Build history of the part. All positions in model axes, mm. A direction names the side the tool comes from. Give positions to 0.01 mm unless a question says otherwise; leave off trailing zeros. Order: outer loops, then holes, each group sorted by start corner. A loop starts at its lowest first (then second) coordinate and runs counter-clockwise, first axis right, second up. Notation, with made-up numbers: (79.5, -23) - (96.5, -23) arc R10 cw to (96.5, -9) - close; hole circle Ø7 at (62.25, 40). An arc over 180 degrees is marked (long way). Use a Markdown table: item, result. Add a question column.
(1) Flat gauge pins, fed straight in: pin 1 (4 mm diameter, centred on x = -3.5, z = -1.5, fed in from +Y); pin 2 (15 mm diameter, centred on x = 0, y = 96.25, fed in from -Z); pin 3 (0.8 mm diameter, centred on x = 5.5, y = -54.5, fed in from -Z). Where does each tip first touch, or does it go through?
(2) Wall check: line 1 (Y direction, x = 5, z = 3.5); line 2 (Y direction, x = 0, z = -0.55); line 3 (X direction, y = -102.25, z = 5). Give the ranges that are in metal, low to high.
(3) Slice it at A-A (y = -31.5). Write the cut outline in (x, z).
(4) Slice it at B-B (y = 93). Write the cut outline in (x, z).
(5) Mould opens along X. For faces 5 (the face through (18, -12, 17)), 6 (the face through (-6.5, 91, 6)), 7 (the face through (0, 113, 0)), 8 (the face through (0, 7, 19)) say: +X half, -X half, draft (parallel to the pull), parting line (faces both ways), or undercut.
(6) Which spindle directions (+Z, -Z, +X, -X, +Y, -Y) get a long thin tool onto all of the face, cutting with end or side? Do faces 1 (the face through (-13.594, -49.031, 15.056)), 2 (the face through (6.5, 91, 6)), 3 (the face through (0, -77, -2)), 4 (the face through (0.266, 70.219, 14.564)). Say none if no direction does.
from build123d import *

# Parameters (mm, degrees)
SKETCH1_W               = 38
SKETCH1_H               = 227.5
SKETCH1_W_2             = 21
SKETCH1_H_2             = 41
BOSS_EXTRUDE1_DEPTH     = 11
SKETCH3_R               = 1.3
CUT_EXTRUDE1_DEPTH      = 8
FILLET3_R               = 19
BOSS_EXTRUDE2_DEPTH     = 8
CUT_EXTRUDE2_DEPTH      = 117.880547997
CUT_EXTRUDE2_DEPTH_BACK = 117.880547997
SKETCH7_W               = 32
SKETCH7_H               = 157.5
BOSS_EXTRUDE4_DEPTH     = 8
SKETCH8_W               = 38
SKETCH8_H               = 157.5
BOSS_EXTRUDE5_DEPTH     = 8
BOSS_EXTRUDE10_START    = 2
SKETCH27_R              = 9
BOSS_EXTRUDE10_DEPTH    = 2
SKETCH28_W              = 38
SKETCH28_H              = 27
BOSS_EXTRUDE11_DEPTH    = 20
FILLET4_R               = 19
CUT_EXTRUDE14_DEPTH     = 8
SKETCH30_W              = 13
SKETCH30_H              = 24
CUT_EXTRUDE15_DEPTH     = 11
CUT_EXTRUDE16_REACH     = 138.422
SKETCH31_R              = 6.5
CUT_EXTRUDE17_START     = 65.75
CUT_EXTRUDE17_OUTLINE_W = 38
CUT_EXTRUDE17_OUTLINE_H = 6
CUT_EXTRUDE17_DEPTH     = 68
FILLET5_R               = 12
CUT_EXTRUDE18_DEPTH     = 141.335535414
FILLET7_R               = 5
SKETCH34_R              = 1.5
CUT_EXTRUDE19_DEPTH     = 8
SKETCH35_R              = 1.1
CUT_EXTRUDE20_DEPTH     = 8
FILLET8_R               = 8
SKETCH36_W              = 21
SKETCH36_H              = 40
CUT_EXTRUDE21_DEPTH     = 2


# Read off the part's stored shape, not the designer's step: Cut-Extrude17
# Some blends are built 0.0001 mm under size
with BuildPart() as part:
    # Sketch1 → Boss-Extrude1 (new body)
    with BuildSketch(Plane.XY):
        Rectangle(SKETCH1_W, SKETCH1_H)
        with Locations((0, -78.25)):
            Rectangle(SKETCH1_W_2, SKETCH1_H_2, mode=Mode.SUBTRACT)
    extrude(amount=BOSS_EXTRUDE1_DEPTH)

    # Sketch3 → Cut-Extrude1 (cut)
    with BuildSketch(Plane.XY.offset(10)):
        with Locations((-5, -54.25)):
            Circle(SKETCH3_R)
        with Locations((5, -54.25)):
            Circle(SKETCH3_R)
        with Locations((5, -102.25)):
            Circle(SKETCH3_R)
        with Locations((-5, -102.25)):
            Circle(SKETCH3_R)
    extrude(amount=-CUT_EXTRUDE1_DEPTH, mode=Mode.SUBTRACT)

    # Fillet3
    fillet3_edges = [part.edges().sort_by_distance(p)[0] for p in [
        (19, -113.75, 5.5),
        (-19, -113.75, 5.5),
    ]]
    fillet(fillet3_edges, radius=FILLET3_R - 0.0001)  # a hair under: the kernel refuses the full size

    # Sketch4 → Boss-Extrude2 (add)
    with BuildSketch(Plane.XY.offset(11)):
        with BuildLine():
            Line((19, -94.75), (19, 113.75))
            Line((19, 113.75), (-19, 113.75))
            Line((-19, 113.75), (-19, -94.75))
            ThreePointArc((-19, -94.75), (-13.435028843, -108.185028843), (0, -113.75))
            ThreePointArc((0, -113.75), (13.435028843, -108.185028843), (19, -94.75))
        make_face()
        with BuildLine():
            Line((16, -94.75), (16, 110.75))
            Line((16, 110.75), (-16, 110.75))
            Line((-16, 110.75), (-16, -94.75))
            ThreePointArc((-16, -94.75), (-11.313708499, -106.063708499), (0, -110.75))
            ThreePointArc((0, -110.75), (11.313708499, -106.063708499), (16, -94.75))
        make_face(mode=Mode.SUBTRACT)
    extrude(amount=BOSS_EXTRUDE2_DEPTH)

    # Sketch6 → Cut-Extrude2 (cut, two sides: drawn at the far end of the back side and taken through both)
    with BuildSketch(Plane(origin=(0, 0, 0), x_dir=(0, 0, -1), z_dir=(1, 0, 0)).offset(-CUT_EXTRUDE2_DEPTH_BACK)):
        Polygon((-13, -113.75), (-16, -88.75), (-19, -73.75), (-19, -113.75), align=None)
    extrude(amount=CUT_EXTRUDE2_DEPTH + CUT_EXTRUDE2_DEPTH_BACK, mode=Mode.SUBTRACT)

    # Sketch7 → Boss-Extrude4 (add)
    with BuildSketch(Plane.XY.offset(11)):
        with Locations((0, 32)):
            Rectangle(SKETCH7_W, SKETCH7_H)
    extrude(amount=BOSS_EXTRUDE4_DEPTH)

    # Sketch8 → Boss-Extrude5 (add)
    with BuildSketch(Plane(origin=(0, 0, 0), x_dir=(-1, 0, 0), z_dir=(0, 0, -1))):
        with Locations((0, 35)):
            Rectangle(SKETCH8_W, SKETCH8_H)
    extrude(amount=BOSS_EXTRUDE5_DEPTH)

    # Sketch27 → Boss-Extrude10 (add)
    with BuildSketch(Plane(origin=(0, 0, 0), x_dir=(-1, 0, 0), z_dir=(0, 0, -1)).offset(BOSS_EXTRUDE10_START)):
        with BuildLine():
            Line((19, -94.75), (19, -43.75))
            Line((19, -43.75), (-19, -43.75))
            Line((-19, -43.75), (-19, -94.75))
            ThreePointArc((-19, -94.75), (-13.435028843, -108.185028843), (0, -113.75))
            ThreePointArc((0, -113.75), (13.435028843, -108.185028843), (19, -94.75))
        make_face()
        with Locations((0, -88.5)):
            Circle(SKETCH27_R, mode=Mode.SUBTRACT)
    extrude(amount=-BOSS_EXTRUDE10_DEPTH)

    # Sketch28 → Boss-Extrude11 (add)
    with BuildSketch(Plane(origin=(0, 113.75, 0), x_dir=(1, 0, 0), z_dir=(0, 1, 0))):
        with Locations((0, -5.5)):
            Rectangle(SKETCH28_W, SKETCH28_H)
    extrude(amount=BOSS_EXTRUDE11_DEPTH)

    # Fillet4
    fillet4_edges = [part.edges().sort_by_distance(p)[0] for p in [
        (-19, 133.75, 5.5),
        (19, 133.75, 5.5),
    ]]
    fillet(fillet4_edges, radius=FILLET4_R - 0.0001)  # a hair under: the kernel refuses the full size

    # Sketch29 → Cut-Extrude14 (cut)
    with BuildSketch(Plane(origin=(0, 0, -8), x_dir=(-1, 0, 0), z_dir=(0, 0, -1))):
        with BuildLine():
            Line((16, 66.75), (16, 114.75))
            ThreePointArc((16, 114.75), (11.313708499, 126.063708499), (0, 130.75))
            ThreePointArc((0, 130.75), (-11.313708499, 126.063708499), (-16, 114.75))
            Line((-16, 114.75), (-16, 66.75))
            Line((-16, 66.75), (16, 66.75))
        make_face()
    extrude(amount=-CUT_EXTRUDE14_DEPTH, mode=Mode.SUBTRACT)

    # Sketch30 → Cut-Extrude15 (cut)
    with BuildSketch(Plane(origin=(0, 0, 0), x_dir=(-1, 0, 0), z_dir=(0, 0, -1))):
        with Locations((0, 90.75)):
            Rectangle(SKETCH30_W, SKETCH30_H)
    extrude(amount=-CUT_EXTRUDE15_DEPTH, mode=Mode.SUBTRACT)

    # Sketch31 → Cut-Extrude16 (cut, up to next)
    with BuildSketch(Plane(origin=(0, 0, 11), x_dir=(-1, 0, 0), z_dir=(0, 0, -1)), mode=Mode.PRIVATE) as cut_extrude16_sk1:
        with Locations(Location((0, 96.25, 0), (0, 0, 180))):
            Circle(SKETCH31_R)
    cut_extrude16_tool1 = extrude(cut_extrude16_sk1.sketch, amount=-CUT_EXTRUDE16_REACH, mode=Mode.PRIVATE) & part.part
    add(cut_extrude16_tool1.solids().sort_by_distance((0, 96.25, 11))[0], mode=Mode.SUBTRACT)

    # Cut-Extrude17 outline → Cut-Extrude17 (cut)
    with BuildSketch(Plane(origin=(0, 0, 0), x_dir=(1, 0, 0), z_dir=(0, 1, 0)).offset(CUT_EXTRUDE17_START)):
        with Locations((0, -16)):
            Rectangle(CUT_EXTRUDE17_OUTLINE_W, CUT_EXTRUDE17_OUTLINE_H)
    extrude(amount=CUT_EXTRUDE17_DEPTH, mode=Mode.SUBTRACT)

    # Fillet5
    # the kernel refuses this fillet: 12 mm, written as the material it adds along each edge
    with BuildSketch(Plane(origin=(-19, -43.75, -2), x_dir=(0, 0, -1), z_dir=(1, 0, 0))) as fillet5_piece_1:
        with BuildLine():
            CenterArc((12, -10.392304845), FILLET5_R, 120, 60)
            Line((0, -10.392304845), (-0.24, -10.392304845))
            Line((-0.24, -10.392304845), (-0.24, 0))
            Line((-0.24, 0), (0, 0.24))
            ThreePointArc((0, 0.24), (3, 0.24), (5.88, 0.207846097))
            Line((5.88, 0.207846097), (6, 0))
        make_face()
    extrude(amount=38)
    with BuildSketch(Plane(origin=(19, 65.75, 13), x_dir=(0, 0, 1), z_dir=(-1, 0, 0))) as fillet5_piece_2:
        with BuildLine():
            CenterArc((12, 10.392304845), FILLET5_R, 180, 60)
            Line((0, 10.392304845), (-0.24, 10.392304845))
            Line((-0.24, 10.392304845), (-0.24, 0))
            Line((-0.24, 0), (0, -0.24))
            ThreePointArc((0, -0.24), (3, -0.24), (5.88, -0.207846097))
            Line((5.88, -0.207846097), (6, 0))
        make_face()
    extrude(amount=38)

    # Sketch33 → Cut-Extrude18 (cut, through all)
    with BuildSketch(Plane(origin=(19, 0, 0), x_dir=(0, 0, -1), z_dir=(1, 0, 0))):
        Polygon((2, 133.75), (8, 93.75), (8, 133.75), align=None)
    extrude(amount=-CUT_EXTRUDE18_DEPTH, mode=Mode.SUBTRACT)

    # Fillet7
    # the kernel refuses this fillet: 5 mm, written as the material it takes off along each edge
    with BuildSketch(Plane(origin=(-19, 123.75, -8), x_dir=(0, 0, 1), z_dir=(0, -1, 0)), Plane(origin=(19, -73.75, -8), x_dir=(0, 0, 1), z_dir=(0, 1, 0))) as fillet7_piece_1:
        with BuildLine():
            CenterArc((FILLET7_R, -FILLET7_R), FILLET7_R, 90, 90)
            Line((0, -FILLET7_R), (-FILLET7_R * 0.02, -FILLET7_R))
            Line((-FILLET7_R * 0.02, -FILLET7_R), (-FILLET7_R * 0.02, FILLET7_R * 0.02))
            Line((-FILLET7_R * 0.02, FILLET7_R * 0.02), (FILLET7_R, FILLET7_R * 0.02))
            Line((FILLET7_R, FILLET7_R * 0.02), (FILLET7_R, 0))
        make_face()
    extrude(amount=197.5, mode=Mode.SUBTRACT)
    with BuildSketch(Plane(origin=(-19, -103.75, 19), x_dir=(1, 0, 0), z_dir=(0, 1, 0)), Plane(origin=(19, 95.75, 19), x_dir=(-1, 0, 0), z_dir=(0, -1, 0))) as fillet7_piece_2:
        with BuildLine():
            CenterArc((FILLET7_R, FILLET7_R), FILLET7_R, 180, 90)
            Line((0, FILLET7_R), (-FILLET7_R * 0.02, FILLET7_R))
            Line((-FILLET7_R * 0.02, FILLET7_R), (-FILLET7_R * 0.02, -FILLET7_R * 0.02))
            Line((-FILLET7_R * 0.02, -FILLET7_R * 0.02), (FILLET7_R, -FILLET7_R * 0.02))
            Line((FILLET7_R, -FILLET7_R * 0.02), (FILLET7_R, 0))
        make_face()
    extrude(amount=199.5, mode=Mode.SUBTRACT)

    # Sketch34 → Cut-Extrude19 (cut)
    with BuildSketch(Plane(origin=(0, 0, 0), x_dir=(-1, 0, 0), z_dir=(0, 0, -1))):
        with Locations((0, 105.75)):
            Circle(SKETCH34_R)
        with Locations((0, 75.75)):
            Circle(SKETCH34_R)
    extrude(amount=-CUT_EXTRUDE19_DEPTH, mode=Mode.SUBTRACT)

    # Sketch35 → Cut-Extrude20 (cut)
    with BuildSketch(Plane.XY.offset(11)):
        with Locations((-5, -54.25)):
            Circle(SKETCH35_R)
        with Locations((5, -54.25)):
            Circle(SKETCH35_R)
        with Locations((5, -102.25)):
            Circle(SKETCH35_R)
        with Locations((-5, -102.25)):
            Circle(SKETCH35_R)
    extrude(amount=-CUT_EXTRUDE20_DEPTH, mode=Mode.SUBTRACT)

    # Fillet8
    fillet8_edges = [part.edges().sort_by_distance(p)[0] for p in [
        (-16, -46.75, 14.791287847),
        (16, -46.75, 14.791287847),
        (16, 66.75, -3.791287847),
        (-16, 66.75, -3.791287847),
    ]]
    fillet(fillet8_edges, radius=FILLET8_R)

    # Sketch36 → Cut-Extrude21 (cut)
    with BuildSketch(Plane(origin=(0, 0, 0), x_dir=(-1, 0, 0), z_dir=(0, 0, -1))):
        with Locations((0, 90.75)):
            Rectangle(SKETCH36_W, SKETCH36_H)
    extrude(amount=-CUT_EXTRUDE21_DEPTH, mode=Mode.SUBTRACT)


solid = part.part
Solution:
| question | item | result |
|---|---|---|
| 1 | pin 1 | y = 133.69 |
| 1 | pin 2 | z = 2 |
| 1 | pin 3 | z = -2 |
| 2 | line 1 | -113.08 to -103.55, -100.95 to -98.75, -57.75 to -55.55, -52.95 to 78.75, 102.75 to 133.08 |
| 2 | line 2 | -113.75 to -97.5, -79.5 to 66.75, 130.75 to 133.75 |
| 2 | line 3 | -17.46 to -6.3, -3.7 to 3.7, 6.3 to 17.46 |
| 3 | outline | (-19, -3) arc R5 ccw to (-14, -8) - (14, -8) arc R5 ccw to (19, -3) - (19, 14) arc R5 ccw to (14, 19) - (-14, 19) arc R5 ccw to (-19, 14) - close |
| 4 | outline | (-19, -3) arc R5 ccw to (-16, -7.58) - (-16, 0) - (-10.5, 0) - (-10.5, 2) - (-6.5, 2) - (-6.5, 11) - (-5.63, 11) - (-5.63, 13) - (-19, 13) - close; (5.63, 11) - (6.5, 11) - (6.5, 2) - (10.5, 2) - (10.5, 0) - (16, 0) - (16, -7.58) arc R5 ccw to (19, -3) - (19, 13) - (5.63, 13) - close |
| 5 | face 5 | +X half |
| 5 | face 6 | undercut |
| 5 | face 7 | undercut |
| 5 | face 8 | draft |
| 6 | face 1 | +Z |
| 6 | face 2 | -Z |
| 6 | face 3 | -Z, +X, -X, -Y |
| 6 | face 4 | +Z, +X, -X, +Y |
